Here's how the part is built. I have some questions about the finished solid (model axes, mm). A direction names the side the tool comes from. Round coordinates to 2 decimals unless told otherwise and drop trailing zeros. Order: outer loops, then holes, each group sorted by start corner. A loop starts at its lowest first (then second) coordinate and runs counter-clockwise, first axis right, second up. Notation, with made-up numbers: (79, 36.25) - (88, 36.25) arc R38 ccw to (88, 74.25) - close; hole circle Ø11 at (84.5, 70). An arc over 180 degrees is marked (long way). Answer as a JSON object with one key per item and string values.
```python
from build123d import *

# Parameters (mm, degrees)
SKETCH1_R           = 75
BOSS_EXTRUDE1_DEPTH = 50
FILLET1_R           = 10
SKETCH4_R           = 17.5
CUT_EXTRUDE1_DEPTH  = 51.0000001


with BuildPart() as part:
    # Sketch1 → Boss-Extrude1 (new body)
    with BuildSketch(Plane.XY):
        Circle(SKETCH1_R)
        with BuildLine():
            Line((0, 30), (0, 60))
            ThreePointArc((0, 60), (-13.351256037, 58.495674731), (-26.033024347, 54.058132074))
            Line((-26.033024347, 54.058132074), (-13.016512174, 27.029066037))
            ThreePointArc((-13.016512174, 27.029066037), (-6.675628019, 29.247837365), (0, 30))
        make_face(mode=Mode.SUBTRACT)
        with BuildLine():
            Line((13.016512174, 27.029066037), (26.033024347, 54.058132074))
            ThreePointArc((26.033024347, 54.058132074), (37.409388112, 46.909888948), (46.909888948, 37.409388112))
            Line((46.909888948, 37.409388112), (23.454944474, 18.704694056))
            ThreePointArc((23.454944474, 18.704694056), (18.704694056, 23.454944474), (13.016512174, 27.029066037))
        make_face(mode=Mode.SUBTRACT)
        with BuildLine():
            Line((29.247837365, 6.675628019), (58.495674731, 13.351256037))
            ThreePointArc((58.495674731, 13.351256037), (60, 0), (58.495674731, -13.351256037))
            Line((58.495674731, -13.351256037), (29.247837365, -6.675628019))
            ThreePointArc((29.247837365, -6.675628019), (30, 0), (29.247837365, 6.675628019))
        make_face(mode=Mode.SUBTRACT)
        with BuildLine():
            Line((23.454944474, -18.704694056), (46.909888948, -37.409388112))
            ThreePointArc((46.909888948, -37.409388112), (37.409388112, -46.909888948), (26.033024347, -54.058132074))
            Line((26.033024347, -54.058132074), (13.016512174, -27.029066037))
            ThreePointArc((13.016512174, -27.029066037), (18.704694056, -23.454944474), (23.454944474, -18.704694056))
        make_face(mode=Mode.SUBTRACT)
        with BuildLine():
            Line((0, -30), (0, -60))
            ThreePointArc((0, -60), (-13.351256037, -58.495674731), (-26.033024347, -54.058132074))
            Line((-26.033024347, -54.058132074), (-13.016512174, -27.029066037))
            ThreePointArc((-13.016512174, -27.029066037), (-6.675628019, -29.247837365), (0, -30))
        make_face(mode=Mode.SUBTRACT)
        with BuildLine():
            Line((-23.454944474, -18.704694056), (-46.909888948, -37.409388112))
            ThreePointArc((-46.909888948, -37.409388112), (-54.058132074, -26.033024347), (-58.495674731, -13.351256037))
            Line((-58.495674731, -13.351256037), (-29.247837365, -6.675628019))
            ThreePointArc((-29.247837365, -6.675628019), (-27.029066037, -13.016512174), (-23.454944474, -18.704694056))
        make_face(mode=Mode.SUBTRACT)
        with BuildLine():
            Line((-29.247837365, 6.675628019), (-58.495674731, 13.351256037))
            ThreePointArc((-58.495674731, 13.351256037), (-54.058132074, 26.033024347), (-46.909888948, 37.409388112))
            Line((-46.909888948, 37.409388112), (-23.454944474, 18.704694056))
            ThreePointArc((-23.454944474, 18.704694056), (-27.029066037, 13.016512174), (-29.247837365, 6.675628019))
        make_face(mode=Mode.SUBTRACT)
    extrude(amount=-BOSS_EXTRUDE1_DEPTH)

    # Fillet1
    fillet1_edges = [part.edges().sort_by_distance(p)[0] for p in [
        (-75, 0, 0),
        (-75, 0, -50),
    ]]
    fillet(fillet1_edges, radius=FILLET1_R)

    # Sketch4 → Cut-Extrude1 (cut, through all)
    with BuildSketch(Plane.XY):
        Circle(SKETCH4_R)
    extrude(amount=-CUT_EXTRUDE1_DEPTH, mode=Mode.SUBTRACT)


solid = part.part
```
1. If I drill on L1, parallel to Y at x = -24, z = -30.5; L2, parallel to X at y = -38.5, z = -37.5; L3, parallel to X at y = 13.5, z = -11 (3 decimals), over which ranges is the centre line in solid material (lowest first)? Write a range as [from, to].
Responses:
{"L1": "[-71.06, -54.99], [-49.84, -19.14], [-18, 18], [19.14, 49.84], [54.99, 71.06]", "L2": "[-64.36, -18.54], [0, 18.54], [46.02, 64.36]", "L3": "[-73.775, -58.462], [-26.791, -11.136], [11.136, 73.775]"}
2. Imagine slicing it at B-B (z = -45). Give the number of separate pieces and of enclosed holes in the cut face, plus the area to 3 significant figures.
Responses:
{"separate pieces": "1", "enclosed holes": "8", "area": "11,800 mm2"}
3. Imagine slicing it at A-A (y = 0). List the corners of the cut face in (x, z) for me, plus the area to 3 significant figures.
Responses:
{"outline": "(-75, -40) arc R10 ccw to (-65, -50) - (-17.5, -50) - (-17.5, 0) - (-65, 0) arc R10 ccw to (-75, -10) - close; (17.5, -50) - (30, -50) - (30, 0) - (17.5, 0) - close; (60, -50) - (65, -50) arc R10 ccw to (75, -40) - (75, -10) arc R10 ccw to (65, 0) - (60, 0) - close", "area": "4,160 mm2"}
4. Thinking about a two-plate mould opening in Y: for faces 3 (the face through (14, 15, -50)), 4 (the face through (-43.667, 9.967, -24.65)), which applies, pulls with the +Y half, pulls with the -Y half, needs draft (parallel to the pull), parting line crosses it, or undercut?
Responses:
{"face 3": "needs draft", "face 4": "undercut"}
5. For faces 1 (the face through (14, 15, 0)), 2 (the face through (-13.167, -58.537, -24.65)), which set-ups out of +Z, -Z, +X, -X, +Y, -Y let a thin tool reach every point of the face, with its end or its side?
Responses:
{"face 1": "+Z, +X, -X, +Y, -Y", "face 2": "+Z, -Z"}
6. For P1, Ø4, axis at x = 54, z = -11, coming from the +Y side; P2, Ø12, axis at x = -50.5, z = -17.5, coming from the -Y side; P3, Ø1.5, axis at y = 48, z = -16.5, coming from the -X side, each with a flat end and sliding along its axis, tell me the tip position at first contact or that it passes through.
Responses:
{"P1": "y = 54.05", "P2": "y = -60.37", "P3": "x = -58.24"}
